```python
from build123d import *

# Parameters (mm, degrees)
BODY_DEPTH             = 3
SKETCH5_W              = 25.4
SKETCH5_H              = 28
PROTOBOARD_MOUNT_DEPTH = 10
SKETCH8_R              = 1.55
STAND_OFF_MOUNT_DEPTH  = 10
SKETCH9_R              = 1.55
PHONE_MOUNT_DEPTH      = 10


with BuildPart() as part:
    # Sketch3 → Body (new body)
    with BuildSketch(Plane(origin=(0, 0, 0), x_dir=(1, 0, 0), z_dir=(0, 1, 0))):
        Polygon((-15, -95), (-47, -95), (-47, -15), (-20, 95), (20, 95), (47, -15), (47, -95), (15, -95), (15, 0), (-15, 0), align=None)
    extrude(amount=BODY_DEPTH)

    # Sketch5 → Protoboard Mount (cut)
    with BuildSketch(Plane(origin=(0, 3, 0), x_dir=(1, 0, 0), z_dir=(0, 1, 0))):
        with Locations((0, 39)):
            Rectangle(SKETCH5_W, SKETCH5_H)
    extrude(amount=-PROTOBOARD_MOUNT_DEPTH, mode=Mode.SUBTRACT)

    # Sketch8 → Stand Off Mount (cut)
    with BuildSketch(Plane(origin=(0, 3, 0), x_dir=(1, 0, 0), z_dir=(0, 1, 0))):
        with Locations(Location((-22.5, 39.4, 0), (0, 0, 270))):
            Circle(SKETCH8_R)
        with Locations(Location((22.5, 39.4, 0), (0, 0, 270))):
            Circle(SKETCH8_R)
        with Locations(Location((37.5, -15.6, 0), (0, 0, 270))):
            Circle(SKETCH8_R)
        with Locations(Location((-37.5, -15.6, 0), (0, 0, 270))):
            Circle(SKETCH8_R)
        with Locations(Location((-17.5, -90.6, 0), (0, 0, 270))):
            Circle(SKETCH8_R)
        with Locations(Location((17.5, -90.6, 0), (0, 0, 270))):
            Circle(SKETCH8_R)
    extrude(amount=-STAND_OFF_MOUNT_DEPTH, mode=Mode.SUBTRACT)

    # Sketch9 → Phone Mount (cut)
    with BuildSketch(Plane(origin=(0, 3, 0), x_dir=(1, 0, 0), z_dir=(0, 1, 0))):
        with Locations(Location((-22.5, 10, 0), (0, 0, 270))):
            Circle(SKETCH9_R)
        with Locations(Location((22.5, 10, 0), (0, 0, 270))):
            Circle(SKETCH9_R)
    extrude(amount=-PHONE_MOUNT_DEPTH, mode=Mode.SUBTRACT)


solid = part.part
```
Model file for the job. Use its own axes, mm. Coordinates: 2 decimals unless noted, no trailing zeros. Order: outer loops, then holes, each group sorted by start corner. A loop starts at its lowest first (then second) coordinate and runs counter-clockwise, first axis right, second up. Notation, with made-up numbers: (-29, 37.25) -> (1, 37.25) arc R18 ccw to (1, 61.25) -> close; hole circle Ø7 at (20.5, 25.25). An arc over 180 degrees is marked (long way). Answer as a JSON object with one key per item and string values. Group by question number.
1) Drill centre lines: L1, parallel to X at y = 0.75, z = -39.4; L2, parallel to X at y = 0.9, z = 90.6; L3, parallel to X at y = 0.75, z = -9. Where is each one in solid material? Low to high.
2) Cut at B-B, the plane y = 1.7. Count the separate pieces of the cut face and the enclosed holes in it, then the cut area to 3 significant figures.
3) Cut at A-A, the plane z = 83. Write the cut outline in (x, y).
4) Cut at D-D, the plane x = 29.5. Write the cut outline in (y, z), then the cut area to 3 significant figures.
5) Flat gauge pins, fed straight in: pin 1 (3.5 mm diameter, centred on x = -22.5, z = -39.4, fed in from -Y); pin 2 (1.9 mm diameter, centred on x = 37.5, z = 15.6, fed in from -Y); pin 3 (0.9 mm diameter, centred on x = -3, y = 1.5, fed in from +Z). Where does each tip first touch, or does it go through?
6) Cut at C-C, the plane x = 6.5. Write the cut outline in (y, z).
Check values:
{
 "1": {"L1": "x = -33.65 to -24.05, -20.95 to -12.7, 12.7 to 20.95, 24.05 to 33.65", "L2": "x = -47 to -19.05, -15.95 to -15, 15 to 15.95, 19.05 to 47", "L3": "x = -41.11 to -23.68, -21.32 to 21.32, 23.68 to 41.11"},
 "2": {"separate pieces": "1", "enclosed holes": "9", "area": "11,300 mm²"},
 "3": {"outline": "(-47, 0) -> (-15, 0) -> (-15, 3) -> (-47, 3) -> close; (15, 0) -> (47, 0) -> (47, 3) -> (15, 3) -> close"},
 "4": {"outline": "(0, -56.3) -> (3, -56.3) -> (3, 95) -> (0, 95) -> close", "area": "454 mm²"},
 "5": {"pin 1": "stops at y = 0", "pin 2": "passes through", "pin 3": "stops at z = 0"},
 "6": {"outline": "(0, -95) -> (3, -95) -> (3, -53) -> (0, -53) -> close; (0, -25) -> (3, -25) -> (3, 0) -> (0, 0) -> close"}
}
